from build123d import *

# Parameters (mm, degrees)
F0_R          = 63.5
F1_DEPTH      = 63.5
F1_DEPTH_BACK = 63.5
F2_R          = 63.5
F3_DEPTH      = 63.5
F3_DEPTH_BACK = 63.5
F4_R          = 63.5
F5_DEPTH      = 63.5
F5_DEPTH_BACK = 63.5


with BuildPart() as f1:
    # F0 (on Front) → F1 (new body, two sides)
    with BuildSketch(Plane.XZ) as f1_sk:
        Circle(F0_R)
    extrude(amount=F1_DEPTH)
    extrude(f1_sk.sketch, amount=-F1_DEPTH_BACK)

    # F2 (on Top) → F3 (join, two sides)
    with BuildSketch(Plane.XY) as f3_sk:
        Circle(F2_R)
    extrude(amount=F3_DEPTH)
    extrude(f3_sk.sketch, amount=-F3_DEPTH_BACK)

    # F4 (on Right) → F5 (join, two sides)
    with BuildSketch(Plane.YZ) as f5_sk:
        Circle(F4_R)
    extrude(amount=F5_DEPTH)
    extrude(f5_sk.sketch, amount=-F5_DEPTH_BACK)


solid = f1.part
Input: part model. Units: mm. Frame: model coordinates. A direction names the side the tool comes from. Round coordinates to 2 decimals unless told otherwise and drop trailing zeros. Write each loop counter-clockwise with the first axis right and the second up, starting at its lowest first coordinate (ties: lowest second). Pieces come first, ordered by that corner, then holes.
1) Cut plane B-B (x = 47.5). Return the cut outline in (y, z), then the cut area to 3 significant figures.
2) Reachability of faces 1 (the cylindrical face through (57.6, 45.1, 44.7)), 2 (the cylindrical face through (-44.7, 45.1, 57.6)), 3 (the cylindrical face through (44.7, 57.6, -45.1)), 4 (the cylindrical face through (-57.6, -45.1, -44.7)), 5 (the cylindrical face through (44.7, -45.1, -57.6)) from +Z, -Z, +X, -X, +Y, -Y: full face, straight path, thin tool, end or side. Return the list, or none.
3) Ray query, L1, parallel to X at y = -51.5, z = -42; L2, parallel to Y at x = -36, z = -56. Return the intervals inside material, ascending.
4) Cut plane C-C (y = -32). Return the cut outline in (x, z), then the cut area to 3 significant figures.
5) Cut plane A-A (z = -49). Return the cut outline in (x, y).
6) Cut plane D-D (z = -33.5). Return the cut outline in (x, y), then the cut area to 3 significant figures.
Geometry says:
1. outline: (-63.5, -42.14) - (-47.5, -42.14) arc R63.5 ccw to (-42.14, -47.5) - (-42.14, -63.5) - (42.14, -63.5) - (42.14, -47.5) arc R63.5 ccw to (47.5, -42.14) - (63.5, -42.14) - (63.5, 42.14) - (47.5, 42.14) arc R63.5 ccw to (42.14, 47.5) - (42.14, 63.5) - (-42.14, 63.5) - (-42.14, 47.5) arc R63.5 ccw to (-47.5, 42.14) - (-63.5, 42.14) - close
1. area: 14,400 mm2
2. face 1: +Z, +X, +Y
2. face 2: +Z, -X, +Y
2. face 3: -Z, +X, +Y
2. face 4: -Z, -X, -Y
2. face 5: -Z, +X, -Y
3. L1: x = -47.63 to 47.63
3. L2: y = -52.31 to 52.31
4. outline: (-63.5, -54.85) - (-54.85, -54.85) - (-54.85, -63.5) - (54.85, -63.5) - (54.85, -54.85) - (63.5, -54.85) - (63.5, 54.85) - (54.85, 54.85) - (54.85, 63.5) - (-54.85, 63.5) - (-54.85, 54.85) - (-63.5, 54.85) - close
4. area: 15,800 mm2
5. outline: (-63.5, -40.39) - (-49, -40.39) arc R63.5 ccw to (-40.39, -49) - (-40.39, -63.5) - (40.39, -63.5) - (40.39, -49) arc R63.5 ccw to (49, -40.39) - (63.5, -40.39) - (63.5, 40.39) - (49, 40.39) arc R63.5 ccw to (40.39, 49) - (40.39, 63.5) - (-40.39, 63.5) - (-40.39, 49) arc R63.5 ccw to (-49, 40.39) - (-63.5, 40.39) - close
6. outline: (-63.5, -53.94) - (-53.94, -53.94) - (-53.94, -63.5) - (53.94, -63.5) - (53.94, -53.94) - (63.5, -53.94) - (63.5, 53.94) - (53.94, 53.94) - (53.94, 63.5) - (-53.94, 63.5) - (-53.94, 53.94) - (-63.5, 53.94) - close
6. area: 15,800 mm2
